from build123d import *

# Parameters (mm, degrees)
SKETCH1_W               = 180
SKETCH1_H               = 920
BOSS_EXTRUDE1_DEPTH     = 80
FILLET2_R               = 3
SHELL1_START            = -497
SHELL1_OUTLINE_W        = 34
SHELL1_OUTLINE_H        = 74
SHELL1_DEPTH            = 994
SHELL1_2_OUTLINE_W      = 541
SHELL1_2_OUTLINE_H      = 74
SHELL1_2_OUTLINE_W_2    = 186
SHELL1_2_DEPTH          = 34
SHELL1_START_2          = 463
SHELL1_3_OUTLINE_W      = 541
SHELL1_3_OUTLINE_H      = 74
SHELL1_3_OUTLINE_W_2    = 186
SHELL1_3_DEPTH          = 34
CUT_EXTRUDE1_DEPTH      = 1435.351421375
CUT_EXTRUDE1_DEPTH_BACK = 1435.351421375
SKETCH2_W               = 74
SKETCH2_H               = 34


# Read off the part's stored shape, not the designer's step: Shell1
with BuildPart() as part:
    # Sketch1 → Boss-Extrude1 (new body)
    with BuildSketch(Plane.XY):
        Polygon((671, -500), (-671, -500), (-671, -460), (-130, -460), (-130, 460), (-671, 460), (-671, 500), (671, 500), (671, 460), (130, 460), (130, -460), (671, -460), align=None)
        Rectangle(SKETCH1_W, SKETCH1_H, mode=Mode.SUBTRACT)
    extrude(amount=-BOSS_EXTRUDE1_DEPTH)

    # Fillet2
    fillet2_edges = [part.edges().sort_by_distance(p)[0] for p in [
        (-90, 0, 0),
        (0, 460, 0),
        (400.5, 460, 0),
        (0, 500, 0),
        (0, -500, 0),
        (-400.5, -460, 0),
        (-130, 0, 0),
        (400.5, -460, 0),
        (0, -460, 0),
        (90, 0, 0),
        (130, 0, 0),
        (400.5, -460, -80),
        (0, -500, -80),
        (-400.5, -460, -80),
        (0, -460, -80),
        (130, 0, -80),
        (90, 0, -80),
        (-90, 0, -80),
        (-130, 0, -80),
        (-400.5, 460, -80),
        (0, 460, -80),
        (400.5, 460, -80),
        (0, 500, -80),
    ]]
    fillet(fillet2_edges, radius=FILLET2_R)

    # Shell1 outline → Shell1 (cut)
    with BuildSketch(Plane(origin=(0, 0, 0), x_dir=(1, 0, 0), z_dir=(0, 1, 0)).offset(SHELL1_START)):
        with Locations((-110, 40)):
            Rectangle(SHELL1_OUTLINE_W, SHELL1_OUTLINE_H)
        with Locations((110, 40)):
            Rectangle(SHELL1_OUTLINE_W, SHELL1_OUTLINE_H)
    extrude(amount=SHELL1_DEPTH, mode=Mode.SUBTRACT)

    # Shell1 2 outline → Shell1 2 (cut)
    with BuildSketch(Plane(origin=(0, 0, 0), x_dir=(1, 0, 0), z_dir=(0, 1, 0)).offset(SHELL1_START)):
        with Locations((-397.5, 40)):
            Rectangle(SHELL1_2_OUTLINE_W, SHELL1_2_OUTLINE_H)
        with Locations((0, 40)):
            Rectangle(SHELL1_2_OUTLINE_W_2, SHELL1_2_OUTLINE_H)
        with Locations((397.5, 40)):
            Rectangle(SHELL1_2_OUTLINE_W, SHELL1_2_OUTLINE_H)
    extrude(amount=SHELL1_2_DEPTH, mode=Mode.SUBTRACT)

    # Shell1 3 outline → Shell1 3 (cut)
    with BuildSketch(Plane(origin=(0, 0, 0), x_dir=(1, 0, 0), z_dir=(0, 1, 0)).offset(SHELL1_START_2)):
        with Locations((-397.5, 40)):
            Rectangle(SHELL1_3_OUTLINE_W, SHELL1_3_OUTLINE_H)
        with Locations((0, 40)):
            Rectangle(SHELL1_3_OUTLINE_W_2, SHELL1_3_OUTLINE_H)
        with Locations((397.5, 40)):
            Rectangle(SHELL1_3_OUTLINE_W, SHELL1_3_OUTLINE_H)
    extrude(amount=SHELL1_3_DEPTH, mode=Mode.SUBTRACT)

    # Sketch2 → Cut-Extrude1 (cut, two sides: drawn at the far end of the back side and taken through both)
    with BuildSketch(Plane(origin=(671, 0, 0), x_dir=(0, 0, -1), z_dir=(1, 0, 0)).offset(-CUT_EXTRUDE1_DEPTH_BACK)):
        with Locations((40, 480)):
            Rectangle(SKETCH2_W, SKETCH2_H)
        with Locations((40, -480)):
            Rectangle(SKETCH2_W, SKETCH2_H)
    extrude(amount=CUT_EXTRUDE1_DEPTH + CUT_EXTRUDE1_DEPTH_BACK, mode=Mode.SUBTRACT)


solid = part.part
For this review, take the finished solid that the model builds, in its own axes (mm). A direction names the side the tool comes from. Coordinates: 2 decimals unless noted, no trailing zeros. Write each loop counter-clockwise with the first axis right and the second up, starting at its lowest first coordinate (ties: lowest second). Pieces come first, ordered by that corner, then holes. Notation, with made-up numbers: (16, 30.25) -> (37, 30.25) arc R21 ccw to (37, 54.25) -> close; hole circle Ø3 at (55, 6). An arc over 180 degrees is marked (long way). Write each question's results on one line, items separated by ' | '. Start each with the question number.
1) Consider section D-D (x = 107.5). Write out the cut boundary in (y, z), plus the area to 3 significant figures.
2) Insertion check: pin 1 (3 mm diameter, centred on y = 86, z = -47, fed in from -X). The pin has a flat end and moves straight along its axis. Give the tip position at first contact, or say it passes through.
3) Consider section B-B (x = -367.5). Write out the cut boundary in (y, z), plus the area to 3 significant figures.
4) The part is to be moulded in two halves that separate along Z. For faces 4 (the face through (-9, -497, -39)), 5 (the face through (-93, -6, -39)), 6 (the face through (103, 2, -80)), 7 (the face through (90, -6, -39)), say which applies: +Z half, -Z half, draft (parallel to the pull), parting line (faces both ways), or undercut.
5) For faces 1 (the face through (96, -39, -3)), 2 (the face through (-130, -6, -39)), 3 (the face through (-403, -463, -39)), list the 3-axis set-ups (+Z, -Z, +X, -X, +Y, -Y) from which the entire face can be reached by the end or side of a thin tool; tool diameter is ignored.
6) Wall thickness on L1, parallel to X at y = 187, z = -20.5; L2, parallel to Y at x = 181, z = -56.5; L3, parallel to Z at x = -117, y = 429.5: over which ranges is each line inside the solid? List them lowest first. Write a range as [from, to].
7) Consider section A-A (y = 297). Write out the cut boundary in (x, z), plus the area to 3 significant figures.
8) Consider section C-C (z = -41). Give the number of separate pieces and of enclosed holes in the cut face, plus the area to 3 significant figures.
Geometry says:
1) outline: (-500, -77) arc R3 ccw to (-497, -80) -> (497, -80) arc R3 ccw to (500, -77) -> (500, -3) arc R3 ccw to (497, 0) -> (-497, 0) arc R3 ccw to (-500, -3) -> close; hole (-497, -77) -> (497, -77) -> (497, -3) -> (-497, -3) -> close | area: 6,440 mm^2
2) pin 1: x = -130
3) outline: (-500, -77) arc R3 ccw to (-497, -80) -> (-463, -80) arc R3 ccw to (-460, -77) -> (-460, -3) arc R3 ccw to (-463, 0) -> (-497, 0) arc R3 ccw to (-500, -3) -> close; (460, -77) arc R3 ccw to (463, -80) -> (497, -80) arc R3 ccw to (500, -77) -> (500, -3) arc R3 ccw to (497, 0) -> (460, 0) -> close; hole (-497, -77) -> (-463, -77) -> (-463, -3) -> (-497, -3) -> close; hole (463, -77) -> (497, -77) -> (497, -3) -> (463, -3) -> close | area: 1,350 mm^2
4) face 4: undercut | face 5: undercut | face 6: -Z half | face 7: draft
5) face 1: none | face 2: +Z, -Z, -X | face 3: +X, -X
6) L1: [-130, -127], [-93, -90], [90, 93], [127, 130] | L2: [-500, -497], [-463, -460], [460, 463], [497, 500] | L3: [-80, -77], [-3, 0]
7) outline: (-130, -77) arc R3 ccw to (-127, -80) -> (-93, -80) arc R3 ccw to (-90, -77) -> (-90, -3) arc R3 ccw to (-93, 0) -> (-127, 0) arc R3 ccw to (-130, -3) -> close; (90, -77) arc R3 ccw to (93, -80) -> (127, -80) arc R3 ccw to (130, -77) -> (130, -3) arc R3 ccw to (127, 0) -> (93, 0) arc R3 ccw to (90, -3) -> close; hole (-127, -77) -> (-93, -77) -> (-93, -3) -> (-127, -3) -> close; hole (93, -77) -> (127, -77) -> (127, -3) -> (93, -3) -> close | area: 1,350 mm^2
8) separate pieces: 5 | enclosed holes: 1 | area: 26,700 mm^2
